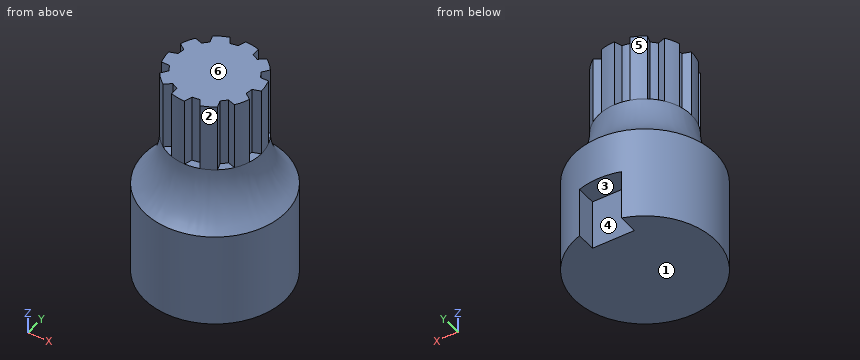
from build123d import *

# Parameters (mm, degrees)
BOSS_EXTRUDE1_DEPTH = 20
CIRPATTERN1_COUNT   = 10
CUT_EXTRUDE1_START  = -11.43
SKETCH3_W           = 9.525
SKETCH3_H           = 5.618681597
CUT_EXTRUDE1_DEPTH  = 11.43


with BuildPart() as part:
    # Sketch1 → Boss-Extrude1 (new body)
    with BuildSketch(Plane.XY):
        with BuildLine():
            Line((0, 10.5), (0, 0))
            Line((0, 0), (6.171745149, 8.494678441))
            Line((6.171745149, 8.494678441), (4.667031658, 7.401440097))
            ThreePointArc((4.667031658, 7.401440097), (3.972416873, 7.796307087), (3.244678441, 8.126165259))
            Line((3.244678441, 8.126165259), (3.244678441, 9.986093421))
            ThreePointArc((3.244678441, 9.986093421), (1.642561883, 10.370727576), (0, 10.5))
        make_face()
    boss_extrude1 = extrude(amount=-BOSS_EXTRUDE1_DEPTH)

    # CirPattern1: Boss-Extrude1 ×10 about axis
    cirpattern1_axis = Axis((0, 0, 0), (0, 0, 1))
    for i in range(1, CIRPATTERN1_COUNT):
        add(boss_extrude1.rotate(cirpattern1_axis, i * 360 / CIRPATTERN1_COUNT))

    # Sketch2 → Revolve1 (revolve)
    with BuildSketch(Plane(origin=(0, 0, 0), x_dir=(0, 0, -1), z_dir=(1, 0, 0))):
        with BuildLine():
            Line((2.355087252, 0), (2.355087252, 8.6))
            Line((2.355087252, 8.6), (15.5, 8.6))
            Line((15.5, 8.6), (15.5, 10.5))
            ThreePointArc((15.5, 10.5), (22.100189391, 11.940495874), (27.5, 16))
            Line((27.5, 16), (48.93, 16))
            Line((48.93, 16), (48.93, 0))
            Line((48.93, 0), (2.355087252, 0))
        make_face()
    revolve(axis=Axis((0, 0, -48.93), (0, 0, 1)))

    # Sketch3 → Cut-Extrude1 (cut)
    with BuildSketch(Plane(origin=(0, 0, -48.93), x_dir=(-1, 0, 0), z_dir=(0, 0, -1)).offset(CUT_EXTRUDE1_START)):
        with Locations((0, 13.639110642)):
            Rectangle(SKETCH3_W, SKETCH3_H)
    extrude(amount=CUT_EXTRUDE1_DEPTH, mode=Mode.SUBTRACT)


solid = part.part
Geometry: final body of the model. Coordinates: model frame, mm. Face numbers are marked on the shaded views. A direction names the side the tool comes from. Coordinates: 2 decimals unless noted, no trailing zeros. Write each loop counter-clockwise with the first axis right and the second up, starting at its lowest first coordinate (ties: lowest second). Pieces come first, ordered by that corner, then holes. Notation, with made-up numbers: (-32, 83) - (-3, 83) arc R25 ccw to (-3, 109) - close; hole circle Ø3 at (-10.75, 37). An arc over 180 degrees is marked (long way). Return JSON: item names as keys, results as strings.
Item 1: Section query A-A (z = -38.5). Output: boundary loops of the cut face in (x, y), and give its area (3 significant figures).
Completed:
{"outline": "(-4.76, 10.83) - (-4.76, 15.27) arc R16 ccw (long way) to (4.76, 15.27) - (4.76, 10.83) - close", "area": "757 mm2"}
Item 2: Pin query (flat end, axial travel): pin 1 Ø4 at (x, z) = (8, -34.5) entering from -Y; pin 2 Ø2 at (x, y) = (-5, -9) entering from +Z; pin 3 Ø1.5 at (y, z) = (-9, -4.5) entering from -X. Return the tip coordinate at first contact, or that it passes through.
Completed:
{"pin 1": "stops at y = -14.83", "pin 2": "stops at z = -15.5", "pin 3": "stops at x = -6.5"}
Item 3: Pull-direction query (X, two-part tool) for the marked faces 4, 5 and 6; classes: +X half, -X half, draft (parallel to the pull), parting line (faces both ways), or undercut.
Completed:
{"face 4": "undercut", "face 5": "-X half", "face 6": "draft"}
Item 4: Section query B-B (z = -32). Output: boundary loops of the cut face in (x, y).
Completed:
{"outline": "circle Ø32 at (0, 0)"}
Item 5: Reachability of the marked faces 1, 2 and 3 from +Z, -Z, +X, -X, +Y, -Y: full face, straight path, thin tool, end or side. Return the list, or none.
Completed:
{"face 1": "-Z, +X, -X, +Y, -Y", "face 2": "+Z, +X, -Y", "face 3": "-Z, +Y"}
Item 6: Section query C-C (z = -23.5). Output: boundary loops of the cut face in (x, y).
Completed:
{"outline": "circle Ø25.34 at (0, 0)"}
Item 7: Line query: L1, parallel to Z at x = -9.5, y = 0.5; L2, parallel to Y at x = -4, z = -42.5; L3, parallel to X at y = 8, z = -28.5. Output: solid intervals per line, ascending.
Completed:
{"L1": "z = -48.93 to -15.5", "L2": "y = -15.49 to 10.83", "L3": "x = -13.86 to 13.86"}
